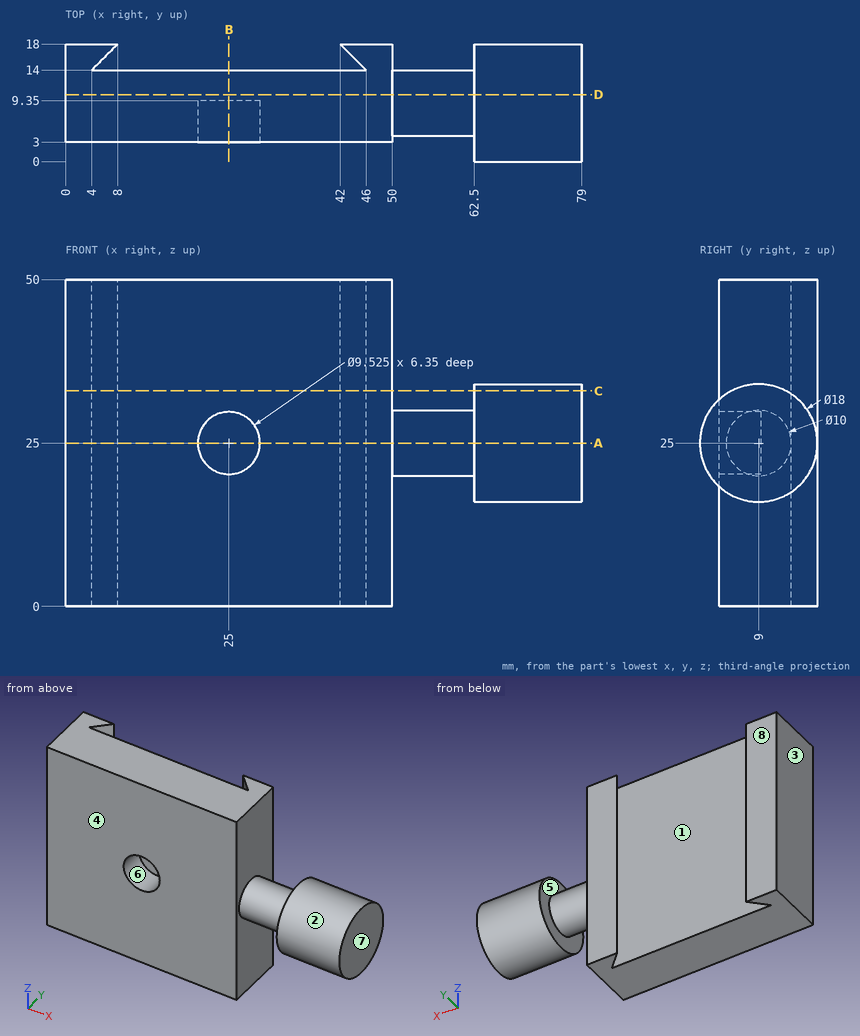
The drawing under review shows one solid part. Ordinate dimensions are in mm from its lowest x, y, z. A direction names the side the tool comes from. Coordinates: 2 decimals unless noted, no trailing zeros. Write each loop counter-clockwise with the first axis right and the second up, starting at its lowest first coordinate (ties: lowest second). Pieces come first, ordered by that corner, then holes. Notation, with made-up numbers: (83, 14) -> (131, 14) arc R7 ccw to (131, 23) -> close; hole circle Ø6 at (55, -21). An arc over 180 degrees is marked (long way). Write each question's results on one line, items separated by ' | '. Start each with the question number.
1) Wall thickness on L1, parallel to Z at x = 25, y = 6; L2, parallel to Y at x = 47.5, z = 8.5; L3, parallel to X at y = 7.75, z = 40: over which ranges is each line inside the solid? List them lowest first. Write a range as [from, to].
2) Consider section B-B (x = 25). Write out the cut boundary in (y, z).
3) For the marked faces 4, 5, 6, 7 and 8, list the 3-axis set-ups (+Z, -Z, +X, -X, +Y, -Y) from which the entire face can be reached by the end or side of a thin tool; tool diameter is ignored.
4) Consider section A-A (z = 25). Write out the cut boundary in (x, y).
5) Insertion check: pin 1 (1 mm diameter, centred on x = 11.5, z = 38, fed in from +Y); pin 2 (10 mm diameter, centred on x = 70.5, z = 7, fed in from +Y); pin 3 (15 mm diameter, centred on x = 30.5, z = 14.5, fed in from -Y). Each pin has a flat end and moves straight along its axis. Give the tip position at first contact, or say it passes through.
6) The part is to be moulded in two halves that separate along X. For the marked faces 1, 2 and 3, say which applies: +X half, -X half, draft (parallel to the pull), parting line (faces both ways), or undercut.
7) Consider section C-C (z = 33). Write out the cut boundary in (x, y), plus the area to 3 significant figures.
8) Consider section D-D (y = 10.25). Write out the cut boundary in (x, z), plus the area to 3 significant figures.
Geometry says:
1) L1: [0, 20.24], [29.76, 50] | L2: [3, 18] | L3: [0, 50]
2) outline: (3, 0) -> (14, 0) -> (14, 50) -> (3, 50) -> (3, 29.76) -> (9.35, 29.76) -> (9.35, 20.24) -> (3, 20.24) -> close
3) face 4: +Z, -Z, -X, -Y | face 5: none | face 6: -Y | face 7: +Z, -Z, +X, +Y, -Y | face 8: +Z, -Z, +X, -X, +Y
4) outline: (0, 3) -> (20.24, 3) -> (20.24, 9.35) -> (29.76, 9.35) -> (29.76, 3) -> (50, 3) -> (50, 4) -> (62.5, 4) -> (62.5, 0) -> (79, 0) -> (79, 18) -> (62.5, 18) -> (62.5, 14) -> (50, 14) -> (50, 18) -> (42, 18) -> (46, 14) -> (4, 14) -> (8, 18) -> (0, 18) -> close
5) pin 1: y = 14 | pin 2: through | pin 3: y = 3
6) face 1: undercut | face 2: draft | face 3: -X half
7) outline: (0, 3) -> (50, 3) -> (50, 18) -> (42, 18) -> (46, 14) -> (4, 14) -> (8, 18) -> (0, 18) -> close; (62.5, 4.88) -> (79, 4.88) -> (79, 13.12) -> (62.5, 13.12) -> close | area: 734 mm^2
8) outline: (0, 0) -> (50, 0) -> (50, 20.16) -> (62.5, 20.16) -> (62.5, 16.09) -> (79, 16.09) -> (79, 33.91) -> (62.5, 33.91) -> (62.5, 29.84) -> (50, 29.84) -> (50, 50) -> (0, 50) -> close | area: 2,920 mm^2
